from build123d import *

# Parameters (mm, degrees)
F0_R      = 11.5
F1_DEPTH  = 23
F2_R      = 8.5
F3_DEPTH  = 3
F4_R      = 3
F5_DEPTH  = 1
F6_R      = 0.5
F7_DEPTH  = 6
F8_R      = 3.5
F9_DEPTH  = 1
F10_R     = 0.5
F11_DEPTH = 0.5
F12_W     = 0.25
F12_H     = 3
F13_DEPTH = 5


with BuildPart() as f1:
    # F0 (on Top) → F1 (new body)
    with BuildSketch(Plane.XY):
        Circle(F0_R)
    extrude(amount=F1_DEPTH)

    # F2 (on face) → F3 (join)
    with BuildSketch(Plane.XY.offset(23)):
        Circle(F2_R)
    extrude(amount=F3_DEPTH)

    # F4 (on face) → F5 (join)
    with BuildSketch(Plane.XY.offset(26)):
        Circle(F4_R)
    extrude(amount=F5_DEPTH)

    # F6 (on face) → F7 (join)
    with BuildSketch(Plane.XY.offset(27)):
        Circle(F6_R)
    extrude(amount=F7_DEPTH)

    # F8 (on face) → F9 (join)
    with BuildSketch(Plane(origin=(0, 0, 0), x_dir=(1, 0, 0), z_dir=(0, 0, -1))):
        Circle(F8_R)
    extrude(amount=F9_DEPTH)

    # F10 (on face) → F11 (join)
    with BuildSketch(Plane(origin=(0, 0, -1), x_dir=(1, 0, 0), z_dir=(0, 0, -1))):
        Circle(F10_R)
    extrude(amount=F11_DEPTH)

    # F12 (on face) → F13 (join)
    with BuildSketch(Plane(origin=(0, 0, 0), x_dir=(1, 0, 0), z_dir=(0, 0, -1))):
        with Locations((-7.9, 0)):
            Rectangle(F12_W, F12_H)
        with Locations((9.1, 0)):
            Rectangle(F12_W, F12_H)
    extrude(amount=F13_DEPTH)


solid = f1.part
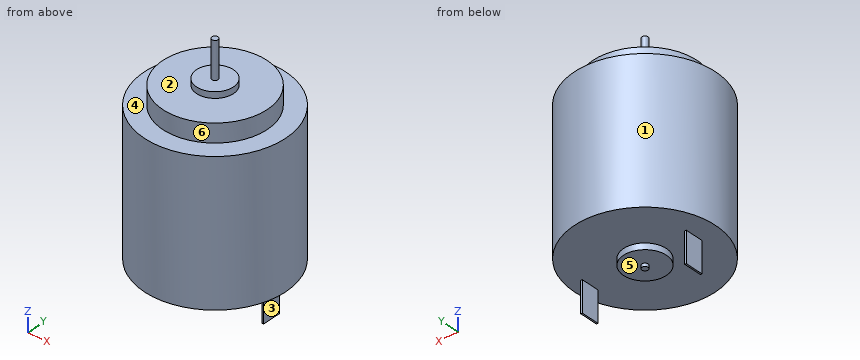
Read the model definition and answer for the solid it produces. Units are mm, in the model's axes. Face numbers are marked on the shaded views. A direction names the side the tool comes from. Give positions to 0.01 mm unless a question says otherwise; leave off trailing zeros. Write each loop counter-clockwise with the first axis right and the second up, starting at its lowest first coordinate (ties: lowest second). Pieces come first, ordered by that corner, then holes. Notation, with made-up numbers: (63, 55) - (93, 55) arc R6 cw to (93, 62) - close; hole circle Ø4 at (-30.5, -7.75). An arc over 180 degrees is marked (long way). Use CSV: the item, a comma, the result in double quotes. Start each with the question number.
Item 1: Flat-ended cylindrical pins translate along their axes: P1, Ø6, axis at y = -3, z = 24, coming from the -X side; P2, Ø11.5, axis at x = -1, y = 1, coming from the -Z side; P3, Ø5, axis at x = -0.5, z = 16.5, coming from the +Y side; P4, Ø1.5, axis at x = -2.5, y = -3.5, coming from the +Z side. Find the tip coordinate at first contact, or state that the pin passes through.
Item 2: The part is cut by section B-B, the plane x = 0. Give the vertices of the cut face in (y, z).
Item 3: The part is cut by section C-C, the plane z = 5. Give the vertices of the cut face in (x, y), and give its area (3 significant figures).
Item 4: The part is cut by section D-D, the plane y = -6.5. Give the vertices of the cut face in (x, z), and give its area (3 significant figures).
Item 5: Consider line 1 (Z direction, x = -3, y = 3); line 2 (Z direction, x = -1.5, y = -0.25); line 3 (X direction, y = 0.25, z = 6.5). Determine where each line is inside the solid, lowest interval first.
Item 6: The mould has two halves that part along X. Classify the marked faces 4, 5 and 6: pulls with the +X half, pulls with the -X half, needs draft (parallel to the pull), parting line crosses it, or undercut.
Item 7: For the marked faces 1, 2 and 3, determine the directions among +Z, -Z, +X, -X, +Y, -Y from which every point of the face is accessible in a straight line to the end or side of a thin tool.
Taken from the geometry:
1,P1,"x = -11.5"
1,P2,"z = -1.5"
1,P3,"y = 11.5"
1,P4,"z = 26"
2,outline,"(-11.5, 0) - (-3.5, 0) - (-3.5, -1) - (-0.5, -1) - (-0.5, -1.5) - (0.5, -1.5) - (0.5, -1) - (3.5, -1) - (3.5, 0) - (11.5, 0) - (11.5, 23) - (8.5, 23) - (8.5, 26) - (3, 26) - (3, 27) - (0.5, 27) - (0.5, 33) - (-0.5, 33) - (-0.5, 27) - (-3, 27) - (-3, 26) - (-8.5, 26) - (-8.5, 23) - (-11.5, 23) - close"
3,outline,"circle Ø23 at (0, 0)"
3,area,"415 mm2"
4,outline,"(-9.49, 0) - (9.49, 0) - (9.49, 23) - (5.48, 23) - (5.48, 26) - (-5.48, 26) - (-5.48, 23) - (-9.49, 23) - close"
4,area,"469 mm2"
5,line 1,"0 to 26"
5,line 2,"-1 to 27"
5,line 3,"-11.5 to 11.5"
6,face 4,"needs draft"
6,face 5,"undercut"
6,face 6,"parting line crosses it"
7,face 1,"+Z, -Z"
7,face 2,"+Z"
7,face 3,"-Z, +X, +Y, -Y"
